Input: part model. Units: mm. Frame: model coordinates. A direction names the side the tool comes from. Coordinates: 2 decimals unless noted, no trailing zeros. Write each loop counter-clockwise with the first axis right and the second up, starting at its lowest first coordinate (ties: lowest second). Pieces come first, ordered by that corner, then holes.
1) Section query B-B (z = 15.5). Output: boundary loops of the cut face in (x, y).
2) Pin query (flat end, axial travel): pin 1 Ø1.5 at (y, z) = (4.5, 12) entering from -X; pin 2 Ø1.5 at (y, z) = (3, 4.5) entering from -X; pin 3 Ø1.6 at (x, y) = (-5, 0) entering from -Z. Return the tip coordinate at first contact, or that it passes through.
3) Section query D-D (z = 5.5). Output: boundary loops of the cut face in (x, y), then the cut area to 3 significant figures.
4) Section query C-C (x = -2). Output: boundary loops of the cut face in (y, z), then the cut area to 3 significant figures.
5) Draft query along Y for faces 4 (the cylindrical face through (6.24, 0.39, 13.07)), 5 (the cylindrical face through (-5.6, -6.64, 4.82)), 6 (the flat face through (-6.5, 0, 5)). Return one class per face: pulls with the +Y half, pulls with the -Y half, needs draft (parallel to the pull), parting line crosses it, or undercut.
6) Set-up query: faces 1 (the cylindrical face through (-3.76, 0.39, 13.07)), 2 (the cylindrical face through (5.6, -6.64, 4.82)), 3 (the flat face through (0, 0, 2)). Return all of +Z, -Z, +X, -X, +Y, -Y with unobstructed straight access to the full face (end or side cutting, diameter ignored); none if empty.
7) Line query: L1, parallel to X at y = 3, z = 9.5; L2, parallel to Z at x = 5.75, y = 1.75; L3, parallel to Y at x = -5, z = 10. Output: solid intervals per line, ascending.
from build123d import *

# Parameters (mm, degrees)
SKETCH_1_W          = 13
SKETCH_1_H          = 15
EXTRUDE_1_DEPTH     = 10
SKETCH_2_W          = 20
SKETCH_2_H          = 15
EXTRUDE_2_DEPTH     = 8
SKETCH_6_R          = 6.25
SKETCH_6_W          = 13
SKETCH_6_H          = 5
CUT_EXTRUDE_3_DEPTH = 2
SKETCH_8_R          = 1.3
CUT_EXTRUDE_5_DEPTH = 10
FILLET_7_R          = 0.5
FILLET_8_R          = 3
FILLET_9_R          = 3
FILLET_10_R         = 0.3


with BuildPart() as part:
    # ｽｹｯﾁ1 → ﾎﾞｽ - 押し出し1 (new body)
    with BuildSketch(Plane.XY):
        Rectangle(SKETCH_1_W, SKETCH_1_H)
    extrude(amount=EXTRUDE_1_DEPTH)

    # ｽｹｯﾁ2 → ﾎﾞｽ - 押し出し2 (add)
    with BuildSketch(Plane.XY.offset(10)):
        Rectangle(SKETCH_2_W, SKETCH_2_H)
    extrude(amount=EXTRUDE_2_DEPTH)

    # ｽｹｯﾁ6 → ｶｯﾄ - 押し出し3 (cut)
    with BuildSketch(Plane(origin=(0, 0, 0), x_dir=(-1, 0, 0), z_dir=(0, 0, -1))):
        Circle(SKETCH_6_R)
        Rectangle(SKETCH_6_W, SKETCH_6_H)
    extrude(amount=-CUT_EXTRUDE_3_DEPTH, mode=Mode.SUBTRACT)

    # ｽｹｯﾁ8 → ｶｯﾄ - 押し出し5 (cut)
    with BuildSketch(Plane.XY.offset(18)):
        with Locations((-5, 0)):
            Circle(SKETCH_8_R)
        with Locations((5, 0)):
            Circle(SKETCH_8_R)
    extrude(amount=-CUT_EXTRUDE_5_DEPTH, mode=Mode.SUBTRACT)

    # ﾌｨﾚｯﾄ7
    fillet_7_edges = [part.edges().sort_by_distance(p)[0] for p in [
        (6.5, 0, 10),
        (-6.5, 0, 10),
    ]]
    fillet(fillet_7_edges, radius=FILLET_7_R)

    # ﾌｨﾚｯﾄ8
    fillet_8_edges = [part.edges().sort_by_distance(p)[0] for p in [
        (10, 0, 10),
        (-10, 0, 10),
    ]]
    fillet(fillet_8_edges, radius=FILLET_8_R - 0.0001)  # a hair under: the kernel refuses the full size

    # ﾌｨﾚｯﾄ9
    fillet_9_edges = [part.edges().sort_by_distance(p)[0] for p in [
        (-10, 7.5, 15.49995),
        (-10, -7.5, 15.49995),
        (10, -7.5, 15.49995),
        (10, 7.5, 15.49995),
        (-6.5, -7.5, 4.75),
        (-6.5, 7.5, 4.75),
        (6.5, 7.5, 4.75),
        (6.5, -7.5, 4.75),
        (-6.646446609, -7.5, 9.853553391),
        (-6.646446609, 7.5, 9.853553391),
        (6.646446609, 7.5, 9.853553391),
        (6.646446609, -7.5, 9.853553391),
        (-9.121349633, 7.5, 10.878650367),
        (9.121349633, 7.5, 10.878650367),
        (-9.121349633, -7.5, 10.878650367),
        (9.121349633, -7.5, 10.878650367),
    ]]
    fillet(fillet_9_edges, radius=FILLET_9_R - 0.0001)  # a hair under: the kernel refuses the full size

    # ﾌｨﾚｯﾄ10
    fillet_10_edges = [part.edges().sort_by_distance(p)[0] for p in [
        (-6.5, 2.5, 1),
        (-5.728219619, 2.5, 1),
        (-6.5, -2.5, 1),
        (5.728219619, -2.5, 1),
        (-5.728219619, -2.5, 1),
        (6.5, -2.5, 1),
        (5.728219619, 2.5, 1),
        (6.5, 2.5, 1),
    ]]
    fillet(fillet_10_edges, radius=FILLET_10_R)


solid = part.part
Answer:
1. outline: (-10, -4.5) arc R3 ccw to (-7, -7.5) - (7, -7.5) arc R3 ccw to (10, -4.5) - (10, 4.5) arc R3 ccw to (7, 7.5) - (-7, 7.5) arc R3 ccw to (-10, 4.5) - close; hole circle Ø2.6 at (-5, 0); hole circle Ø2.6 at (5, 0)
2. pin 1: stops at x = -9.99
2. pin 2: stops at x = -6.5
2. pin 3: stops at z = 2
3. outline: (-6.5, -4.5) arc R3 ccw to (-3.5, -7.5) - (3.5, -7.5) arc R3 ccw to (6.5, -4.5) - (6.5, 4.5) arc R3 ccw to (3.5, 7.5) - (-3.5, 7.5) arc R3 ccw to (-6.5, 4.5) - close
3. area: 187 mm2
4. outline: (-7.5, 0) - (-5.92, 0) - (-5.92, 2) - (5.92, 2) - (5.92, 0) - (7.5, 0) - (7.5, 18) - (-7.5, 18) - close
4. area: 246 mm2
5. face 4: undercut
5. face 5: pulls with the -Y half
5. face 6: needs draft
6. face 1: +Z
6. face 2: -Z, +X, -Y
6. face 3: -Z
7. L1: x = -6.5 to 6.5
7. L2: z = 2 to 18
7. L3: y = -7.13 to -1.3, 1.3 to 7.13
